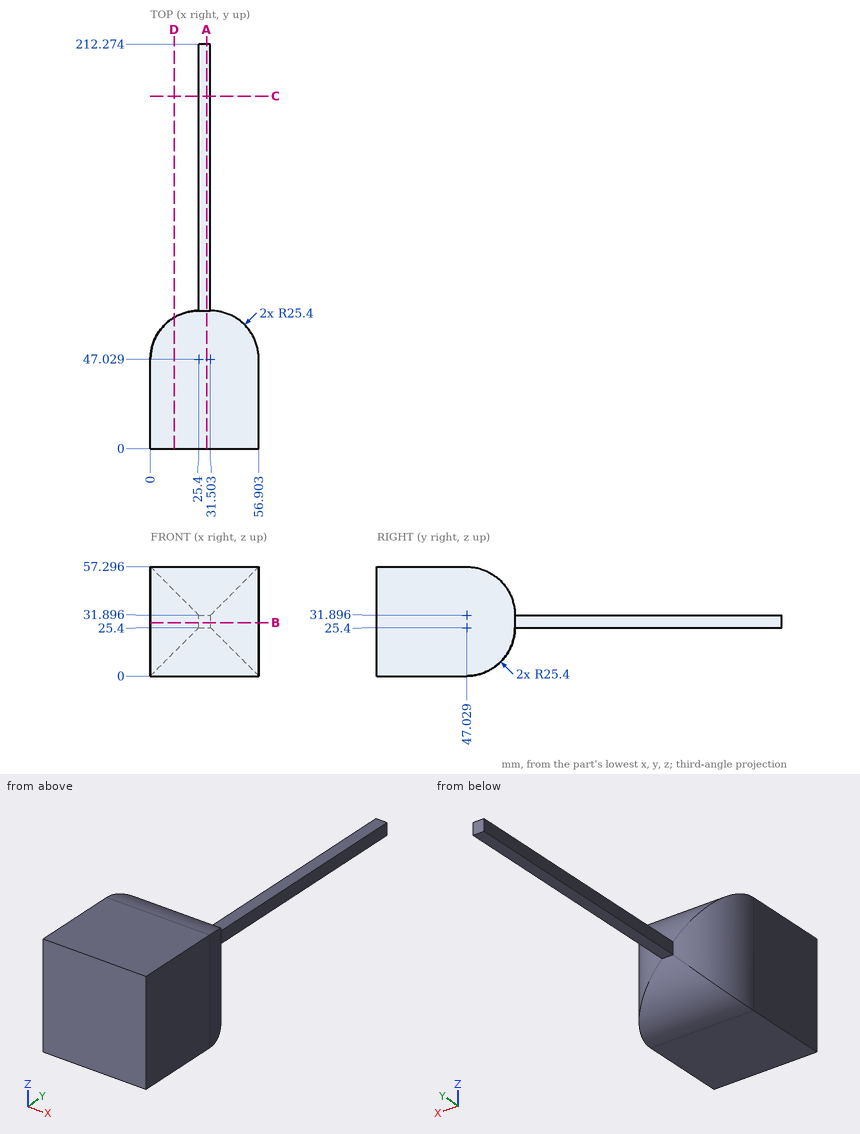
Study the drawing (mm; zero at the part's minimum x, y, z) and answer. Give positions to 0.01 mm unless a question says otherwise; leave off trailing zeros. Loops run counter-clockwise (first coordinate to the right, second up) from the corner with the lowest first, then second, coordinate; pieces in that order, holes last. Notation, with made-up numbers: (77.5, -24) - (135.5, -24) arc R15 ccw to (135.5, -20) - close; hole circle Ø1 at (16.5, 83). An arc over 180 degrees is marked (long way). Use CSV: the item, a comma, the result in double quotes. Start each with the question number.
(1) Find the intervals of material crossed by L1, parallel to Z at x = 25.5, y = 192 (1 decimal); L2, parallel to Y at x = 29.5, z = 25 (1 decimal); L3, parallel to Y at x = 12, z = 16.5 (1 decimal), in increasing order.
(2) Find section C-C, the plane y = 185. Determine the outline of the cut face in (x, z) (1 decimal).
(3) Each of these flat-tipped pins is pushed along its axis until it touches: pin 1 (10 mm diameter, centred on y = 151, z = 34, fed in from -X); pin 2 (7 mm diameter, centred on y = 154.5, z = 29.5, fed in from +X); pin 3 (4 mm diameter, centred on x = 27.5, z = 46.5, fed in from +Y); pin 4 (8 mm diameter, centred on x = 17.5, z = 26.5, fed in from -Y). Where does it stop, or does it pass through?
(4) Find section D-D, the plane x = 12.5. Determine the outline of the cut face in (y, z) (1 decimal).
(5) Find section A-A, the plane x = 29.5. Determine the outline of the cut face in (y, z) (1 decimal), plus the area to 3 significant figures.
(6) Find section B-B, the plane z = 28. Determine the outline of the cut face in (x, y) (1 decimal).
Results found:
1,L1,"25.4 to 31.9"
1,L2,"0 to 72.4"
1,L3,"0 to 68.6"
2,outline,"(25.4, 25.4) - (31.5, 25.4) - (31.5, 31.9) - (25.4, 31.9) - close"
3,pin 1,"x = 25.4"
3,pin 2,"x = 31.5"
3,pin 3,"y = 69.08"
3,pin 4,"y = 0"
4,outline,"(0, 0) - (47, 0) arc R25.4 ccw to (68.9, 12.5) - (68.9, 44.8) arc R25.4 ccw to (47, 57.3) - (0, 57.3) - close"
5,outline,"(0, 0) - (47, 0) arc R25.4 ccw to (72.4, 25.4) - (212.3, 25.4) - (212.3, 31.9) - (72.4, 31.9) arc R25.4 ccw to (47, 57.3) - (0, 57.3) - close"
5,area,"4,780 mm^2"
6,outline,"(0, 0) - (56.9, 0) - (56.9, 47) arc R25.4 ccw to (31.5, 72.4) - (31.5, 212.3) - (25.4, 212.3) - (25.4, 72.4) arc R25.4 ccw to (0, 47) - close"
